Part model, mm, in its own coordinate system. A direction names the side the tool comes from. Give positions to 0.01 mm unless a question says otherwise; leave off trailing zeros. Order: outer loops, then holes, each group sorted by start corner. A loop starts at its lowest first (then second) coordinate and runs counter-clockwise, first axis right, second up. Notation, with made-up numbers: (-21.75, -11) - (16.25, -11) arc R9 ccw to (16.25, -2) - close; hole circle Ø1 at (67, 28.25). An arc over 180 degrees is marked (long way). One line per item, written item: value.
```python
from build123d import *

# Parameters (mm, degrees)
MAIN_PROFILE_DEPTH                             = 50.8
END_ROUNDS_DEPTH                               = 25.4
SKETCH3_W                                      = 3.302
SKETCH3_H                                      = 4.7625
SKETCH3_H_2                                    = 4.1275
LOCATING_FLANGE_DEPTH                          = 53.111155755
BUTTON_POCKETS_DEPTH                           = 3.81
CBORE_FOR_2_SOCKET_HEAD_CAP_SCREW1_D           = 2.4384
CBORE_FOR_2_SOCKET_HEAD_CAP_SCREW1_CBORE_D     = 4.572
CBORE_FOR_2_SOCKET_HEAD_CAP_SCREW1_CBORE_DEPTH = 1.27
F_1_16_0_0625_DIAMETER_HOLE1_D                 = 1.5875


with BuildPart() as part:
    # Sketch1 → Main profile (new body)
    with BuildSketch(Plane(origin=(0, 0, 0), x_dir=(1, 0, 0), z_dir=(0, 1, 0))):
        with BuildLine():
            Line((-4.191328185, 1.27), (5.333671815, 1.27))
            Line((5.333671815, 1.27), (5.333671815, 6.35))
            ThreePointArc((5.333671815, 6.35), (0.571171815, 6.648828143), (-4.191328185, 6.35))
            Line((-4.191328185, 6.35), (-4.191328185, 1.27))
        make_face()
    extrude(amount=MAIN_PROFILE_DEPTH)

    # Sketch2 → End rounds (cut)
    with BuildSketch(Plane.XY.offset(-1.27)):
        with BuildLine():
            Line((-4.191328185, 50.8), (-4.191328185, 46.0375))
            ThreePointArc((-4.191328185, 46.0375), (-2.796424231, 49.405096045), (0.571171815, 50.8))
            Line((0.571171815, 50.8), (-4.191328185, 50.8))
        make_face()
        with BuildLine():
            Line((5.333671815, 50.8), (0.571171815, 50.8))
            ThreePointArc((0.571171815, 50.8), (3.93876786, 49.405096045), (5.333671815, 46.0375))
            Line((5.333671815, 46.0375), (5.333671815, 50.8))
        make_face()
        with BuildLine():
            ThreePointArc((5.333671815, 4.7625), (3.938767861, 1.394903955), (0.571171817, 0))
            Line((0.571171817, 0), (5.333671815, 0))
            Line((5.333671815, 0), (5.333671815, 4.7625))
        make_face()
        with BuildLine():
            ThreePointArc((0.571171817, 0), (-2.79642423, 1.394903954), (-4.191328185, 4.7625))
            Line((-4.191328185, 4.7625), (-4.191328185, 0))
            Line((-4.191328185, 0), (0.571171817, 0))
        make_face()
    extrude(amount=-END_ROUNDS_DEPTH, mode=Mode.SUBTRACT)

    # Sketch3 → Locating Flange (cut, through all)
    with BuildSketch(Plane.ZY.offset(4.191328185)):
        with Locations((-2.921, 2.38125)):
            Rectangle(SKETCH3_W, SKETCH3_H)
        with Locations((-2.921, 6.82625)):
            Rectangle(SKETCH3_W, SKETCH3_H_2)
        with Locations((-2.921, 43.97375)):
            Rectangle(SKETCH3_W, SKETCH3_H_2)
        with Locations((-2.921, 48.41875)):
            Rectangle(SKETCH3_W, SKETCH3_H)
    extrude(amount=-LOCATING_FLANGE_DEPTH, mode=Mode.SUBTRACT)

    # Sketch4 → Button Pockets (cut)
    with BuildSketch(Plane(origin=(0, 0, -6.648828143), x_dir=(-1, 0, 0), z_dir=(0, 0, -1))):
        with BuildLine():
            Line((-2.682671815, 38.735), (1.540328185, 38.735))
            ThreePointArc((1.540328185, 38.735), (2.337237528, 38.404909342), (2.667328185, 37.608))
            Line((2.667328185, 37.608), (2.667328185, 33.385))
            ThreePointArc((2.667328185, 33.385), (2.337237528, 32.588090658), (1.540328185, 32.258))
            Line((1.540328185, 32.258), (-2.682671815, 32.258))
            ThreePointArc((-2.682671815, 32.258), (-3.479581157, 32.588090658), (-3.809671815, 33.385))
            Line((-3.809671815, 33.385), (-3.809671815, 37.608))
            ThreePointArc((-3.809671815, 37.608), (-3.479581157, 38.404909342), (-2.682671815, 38.735))
        make_face()
        with BuildLine():
            Line((-2.682671815, 29.226), (1.540328185, 29.226))
            ThreePointArc((1.540328185, 29.226), (2.337237528, 28.895909342), (2.667328185, 28.099))
            Line((2.667328185, 28.099), (2.667328185, 23.876))
            ThreePointArc((2.667328185, 23.876), (2.337237528, 23.079090658), (1.540328185, 22.749))
            Line((1.540328185, 22.749), (-2.682671815, 22.749))
            ThreePointArc((-2.682671815, 22.749), (-3.479581157, 23.079090658), (-3.809671815, 23.876))
            Line((-3.809671815, 23.876), (-3.809671815, 28.099))
            ThreePointArc((-3.809671815, 28.099), (-3.479581157, 28.895909342), (-2.682671815, 29.226))
        make_face()
        with BuildLine():
            Line((-2.682671815, 18.542), (1.540328185, 18.542))
            ThreePointArc((1.540328185, 18.542), (2.337237528, 18.211909342), (2.667328185, 17.415))
            Line((2.667328185, 17.415), (2.667328185, 13.192))
            ThreePointArc((2.667328185, 13.192), (2.337237528, 12.395090658), (1.540328185, 12.065))
            Line((1.540328185, 12.065), (-2.682671815, 12.065))
            ThreePointArc((-2.682671815, 12.065), (-3.479581157, 12.395090658), (-3.809671815, 13.192))
            Line((-3.809671815, 13.192), (-3.809671815, 17.415))
            ThreePointArc((-3.809671815, 17.415), (-3.479581157, 18.211909342), (-2.682671815, 18.542))
        make_face()
    extrude(amount=-BUTTON_POCKETS_DEPTH, mode=Mode.SUBTRACT)

    # CBORE for #2 Socket Head Cap Screw1 (through all)
    with Locations(Plane(origin=(0, 0, -6.648828143), x_dir=(-1, 0, 0), z_dir=(0, 0, -1))):
        with Locations((-0.571171815, 46.0375), (-0.571171815, 4.7625)):
            CounterBoreHole(CBORE_FOR_2_SOCKET_HEAD_CAP_SCREW1_D / 2, CBORE_FOR_2_SOCKET_HEAD_CAP_SCREW1_CBORE_D / 2, CBORE_FOR_2_SOCKET_HEAD_CAP_SCREW1_CBORE_DEPTH)

    # 1/16 (0.0625) Diameter Hole1 (through all)
    with Locations(Plane.XY.offset(-1.27)):
        with Locations((-1.524328185, 35.4965), (2.666671815, 35.4965), (2.666671815, 25.9875), (-1.524328185, 25.9875), (-1.524328185, 15.3035), (2.666671815, 15.3035)):
            Hole(F_1_16_0_0625_DIAMETER_HOLE1_D / 2)


solid = part.part
```
1) Drop flat-ended pins along their axis: P1, Ø4.5, axis at x = -2, y = 46, coming from the +Z side; P2, Ø1.8, axis at x = 2.67, y = 15.3, coming from the -Z side; P3, Ø1.4, axis at x = 0, y = 45, coming from the -Z side. Give the stop position or say it passes through.
Answer:
P1: stops at z = -4.57
P2: stops at z = -2.84
P3: stops at z = -5.38
2) Wall check: line 1 along Y through (x, z) = (2.75, -3.75); line 2 along Y through (x, z) = (-1.5, -1.7); line 3 along X through (y, z) = (37, -3). Give the ranges that are in metal, low to high. Write a range as [from, to].
Answer:
line 1: y = [8.89, 12.07], [18.54, 22.75], [29.22, 32.26], [38.73, 41.91]
line 2: y = [8.89, 14.51], [16.1, 25.19], [26.78, 34.7], [36.29, 41.91]
line 3: x = [-4.19, -2.67], [3.81, 5.33]
3) Slice it at C-C on z = -1.75. Write the cut outline in (x, y), then the cut area to 3 significant figures.
Answer:
outline: (-4.19, 8.89) - (5.33, 8.89) - (5.33, 41.91) - (-4.19, 41.91) - close; hole circle Ø1.59 at (-1.52, 15.3); hole circle Ø1.59 at (-1.52, 25.99); hole circle Ø1.59 at (-1.52, 35.5); hole circle Ø1.59 at (2.67, 15.3); hole circle Ø1.59 at (2.67, 25.99); hole circle Ø1.59 at (2.67, 35.5)
area: 303 mm2
4) Two-plate mould, pull along X, no slides. Class faces 3 (the face through (4.873, 25.044, -6.405)), 4 (the face through (2.77, 36.283, -2.065)), 5 (the face through (5.334, 25, -4)), 6 (the face through (3.471, 12.386, -4.741)): pulls with the +X half, pulls with the -X half, needs draft (parallel to the pull), parting line crosses it, or undercut.
Answer:
face 3: parting line crosses it
face 4: undercut
face 5: pulls with the +X half
face 6: undercut
5) Slice it at B-B on y = 45.5. Write the cut outline in (x, z), then the cut area to 3 significant figures.
Answer:
outline: (-4.19, -6.35) arc R38.1 ccw to (-1.65, -6.58) - (-1.65, -5.38) - (-0.52, -5.38) - (-0.52, -4.57) - (-4.19, -4.57) - close; (1.67, -5.38) - (2.79, -5.38) - (2.79, -6.58) arc R38.1 ccw to (5.33, -6.35) - (5.33, -4.57) - (1.67, -4.57) - close
area: 11.5 mm2
6) Slice it at A-A on z = -4. Write the cut outline in (x, y) (3 decimals).
Answer:
outline: (-4.191, 8.89) - (5.334, 8.89) - (5.334, 41.91) - (-4.191, 41.91) - close; hole (-2.667, 13.192) arc R1.127 ccw to (-1.54, 12.065) - (2.683, 12.065) arc R1.127 ccw to (3.81, 13.192) - (3.81, 17.415) arc R1.127 ccw to (2.683, 18.542) - (-1.54, 18.542) arc R1.127 ccw to (-2.667, 17.415) - close; hole (-2.667, 23.876) arc R1.127 ccw to (-1.54, 22.749) - (2.683, 22.749) arc R1.127 ccw to (3.81, 23.876) - (3.81, 28.099) arc R1.127 ccw to (2.683, 29.226) - (-1.54, 29.226) arc R1.127 ccw to (-2.667, 28.099) - close; hole (-2.667, 33.385) arc R1.127 ccw to (-1.54, 32.258) - (2.683, 32.258) arc R1.127 ccw to (3.81, 33.385) - (3.81, 37.608) arc R1.127 ccw to (2.683, 38.735) - (-1.54, 38.735) arc R1.127 ccw to (-2.667, 37.608) - close
7) Which spindle directions (+Z, -Z, +X, -X, +Y, -Y) get a long thin tool onto all of the face, cutting with end or side? Do faces 1 (the face through (2.839, 25.213, -2.065)), 2 (the face through (3.488, 38.396, -4.741)). Say none if no direction does.
Answer:
face 1: +Z, -Z
face 2: -Z
8) Slice it at D-D on y = 31. Write the cut outline in (x, z), then the cut area to 3 significant figures.
Answer:
outline: (-4.19, -6.35) arc R38.1 ccw to (5.33, -6.35) - (5.33, -1.27) - (-4.19, -1.27) - close
area: 50.3 mm2
